Part model, mm, in its own coordinate system. Coordinates: 2 decimals unless noted, no trailing zeros. Loops run counter-clockwise (first coordinate to the right, second up) from the corner with the lowest first, then second, coordinate; pieces in that order, holes last. Notation, with made-up numbers: (-23, 21) -> (-1, 21) arc R32 cw to (-1, 55) -> close; hole circle Ø10 at (47.5, 43). An arc over 180 degrees is marked (long way). One line per question, with ' | ' between items. Start each with the question number.
1) Cut at B-B (z = 1.9). Count the separate pieces of the cut face and the enclosed holes in it, plus the area to 3 significant figures.
2) Cut at A-A (x = 20). List the corners of the cut face in (y, z), plus the area to 3 significant figures.
3) Drop flat-ended pins along their axis: pin 1 (1.3 mm diameter, centred on x = 147.5, z = 2.5, fed in from +Y); pin 2 (2 mm diameter, centred on y = 13, z = 3, fed in from +X); pin 3 (3 mm diameter, centred on x = -25.4, y = 7.62, fed in from +Z). Give the stop position or say it passes through.
4) Probe L1, parallel to X at y = 7.62, z = 2.35; L2, parallel to X at y = 83.5, z = 0.9; L3, parallel to X at y = 81, z = 1.6. List the from-to ranges inside material, lowest first. Write a range as from..to.
5) Cut at C-C (y = 34.5). List the corners of the cut face in (x, z), plus the area to 3 significant figures.
Autodesk Inventor part; units mm, degrees
ref_plane "YZ Plane" through (0, 0, 0) normal (1, 0, 0) x (0, 1, 0)
ref_plane "XZ Plane" through (0, 0, 0) normal (0, 1, 0) x (-1, 0, 0)
ref_plane "XY Plane" through (0, 0, 0) normal (0, 0, 1) x (1, 0, 0)
sketch "Sketch1" plane through (0, 0, 0) normal (0, 0, 1) x (1, 0, 0)
  line L0 (0, 105.156) -> (0, -17.526)
  line L1 (-209.804, 0) -> (209.804, 0)
  line L2 (101.6, 25.4) -> (-101.6, 25.4)
  line L3 (-101.6, 25.4) -> (-101.6, 0)
  line L4 (-101.6, 0) -> (101.6, 0)
  line L5 (101.6, 0) -> (101.6, 25.4)
  line L6 (101.6, 25.4) -> (-101.6, 0) construction
  line L7 (-101.6, 25.4) -> (101.6, 0) construction
  line L8 (149.86, 87.63) -> (-149.86, 87.63)
  line L9 (-149.86, 87.63) -> (-149.86, 25.4)
  line L10 (-149.86, 25.4) -> (149.86, 25.4)
  line L11 (149.86, 25.4) -> (149.86, 87.63)
  line L12 (149.86, 87.63) -> (-149.86, 25.4) construction
  line L13 (-149.86, 87.63) -> (149.86, 25.4) construction
  point P0 (0, 0)
  point P1 (0, 12.7)
  point P2 (0, 56.515)
  point P3 (-76.2, 7.62)
  point P4 (-25.4, 7.62)
  point P5 (25.4, 7.62)
  point P6 (76.2, 7.62)
  point P7 (-132.08, 79.8322)
  point P8 (132.08, 79.8322)
  point P9 (0, 79.8322)
  point P10 (-38.1, 79.8322)
  point P11 (38.1, 79.8322)
  dimension "d0" = 203.2
  dimension "d1" = 25.4
  dimension "d2" = 0
  dimension "d5" = 25.4
  dimension "d6" = 50.8
  dimension "d7" = 7.62
  dimension "d8" = 25.4
  dimension "d9" = 50.8
  dimension "d30" = 132.08
  dimension "d31" = 132.08
  dimension "d32" = 79.8322
  dimension "d33" = 87.63
  dimension "d34" = 299.72
  dimension "d62" = 38.1
  dimension "d63" = 38.1
extrude "Extrusion1" add sketch "Sketch1" along normal blind 4.4958
hole "Hole1" at (-76.2, 7.62, 0) at (-25.4, 7.62, 0) at (25.4, 7.62, 0) at (76.2, 7.62, 0) direction (0, 0, 1) diameter 3.1242 end through all
hole "Hole2" at (-132.08, 79.8322, 0) at (132.08, 79.8322, 0) at (0, 79.8322, 0) at (-38.1, 79.8322, 0) at (38.1, 79.8322, 0) direction (0, 0, 1) diameter 3.81 end through all
sketch "Sketch2" plane through (0, 0, 0) normal (0, 0, 1) x (1, 0, 0)
  circle A0 centre (132.08, 79.8322) radius 1.905
  circle A1 centre (-132.08, 79.8322) radius 1.905
  circle A2 centre (0, 79.8322) radius 1.905
  circle A3 centre (25.4, 7.62) radius 1.5621
  circle A4 centre (-76.2, 7.62) radius 1.5621
  circle A5 centre (-25.4, 7.62) radius 1.5621
  circle A6 centre (76.2, 7.62) radius 1.5621
  line L0 (-101.6, 25.4) -> (-101.6, 0)
  line L1 (-101.6, 0) -> (101.6, 0)
  line L2 (101.6, 0) -> (101.6, 25.4)
  line L3 (101.6, 25.4) -> (149.86, 25.4)
  line L4 (149.86, 25.4) -> (149.86, 87.63)
  line L5 (149.86, 87.63) -> (-149.86, 87.63)
  line L6 (-149.86, 87.63) -> (-149.86, 25.4)
  line L7 (-149.86, 25.4) -> (-101.6, 25.4)
  line L8 (-149.86, 87.63) -> (-137.16, 87.63)
  line L9 (-137.16, 87.63) -> (-137.16, 76.2)
  line L10 (-137.16, 76.2) -> (-149.86, 76.2)
  line L11 (-149.86, 76.2) -> (-149.86, 87.63)
  line L12 (149.86, 87.63) -> (137.16, 87.63)
  line L13 (137.16, 87.63) -> (137.16, 76.2)
  line L14 (137.16, 76.2) -> (149.86, 76.2)
  line L15 (149.86, 76.2) -> (149.86, 87.63)
  line L16 (-149.86, 87.63) -> (-149.2523, 87.63)
  line L17 (-149.2523, 87.63) -> (-151.5626, 87.63)
  line L18 (-151.5626, 87.63) -> (-149.86, 87.63)
  point P0 (0, 0)
  point P1 (-144.78, 67.945)
  point P2 (144.78, 67.945)
  point P3 (-138.43, 67.945)
  point P4 (138.43, 67.945)
  dimension "d35" = 11.43
  dimension "d36" = 12.7
  dimension "d39" = 8.255
  dimension "d40" = 5.08
  dimension "d41" = 5.08
  dimension "d64" = 6.35
  dimension "d65" = 6.35
extrude "Extrusion2" cut sketch "Sketch2" along normal up to next contours L6 L5 L9 L10 | L14 L13 L5 L4
hole "Hole3" at (-144.78, 67.945, 0) at (144.78, 67.945, 0) at (-138.43, 67.945, 0) at (138.43, 67.945, 0) direction (0, 0, 1) diameter 3.81 end through all
sketch "Sketch3" plane through (0, 0, 0) normal (0, 0, 1) x (1, 0, 0)
  line L0 (0, 105.156) -> (0, -17.526)
  line L1 (-209.804, 0) -> (209.804, 0)
  line L2 (137.16, 87.63) -> (-137.16, 87.63)
  line L3 (63.5, 83.058) -> (-63.5, 83.058)
  line L4 (-63.5, 83.058) -> (-63.5, 87.63)
  line L5 (-63.5, 87.63) -> (63.5, 87.63)
  line L6 (63.5, 87.63) -> (63.5, 83.058)
  line L7 (63.5, 83.058) -> (-63.5, 87.63) construction
  line L8 (-63.5, 83.058) -> (63.5, 87.63) construction
  point P0 (0, 0)
  point P1 (0, 85.344)
  dimension "d49" = 4.572
  dimension "d50" = 127
extrude "Extrusion3" cut sketch "Sketch3" along normal up to next
fillet "Fillet1" radius 6.35 2 edges at (-137.16, 76.2, 2.2479) (137.16, 76.2, 2.2479)
chamfer "Chamfer1" distance 38.1 angle 30 1 edges at (149.86, 25.4, 2.2479) measured on face at (117.6867, 25.4, 1.4986)
chamfer "Chamfer2" distance 38.1 angle 30 1 edges at (-149.86, 25.4, 2.2479) measured on face at (-133.7733, 25.4, 1.4986)
fillet "Fillet2" radius 12.7 4 edges at (-149.86, 47.397, 2.2479) (-111.76, 25.4, 2.2479) (111.76, 25.4, 2.2479) (149.86, 47.397, 2.2479)
fillet "Fillet3" radius 6.35 2 edges at (-101.6, 25.4, 2.2479) (101.6, 25.4, 2.2479)
properties material "DELRIN 100, BLACK (EXTRUDED)"
Reported:
1) separate pieces: 1 | enclosed holes: 13 | area: 22,000 mm²
2) outline: (0, 0) -> (83.06, 0) -> (83.06, 4.5) -> (0, 4.5) -> close | area: 373 mm²
3) pin 1: stops at y = 76.2 | pin 2: stops at x = 101.6 | pin 3: passes through
4) L1: x = -101.6..-77.76, -74.64..-26.96, -23.84..23.84, 26.96..74.64, 77.76..101.6 | L2: x = -137.16..-63.5, 63.5..137.16 | L3: x = -137.35..-133.59, -130.57..-39.61, -36.59..-1.51, 1.51..36.59, 39.61..130.57, 133.59..137.35
5) outline: (-127.52, 0) -> (127.52, 0) -> (127.52, 4.5) -> (-127.52, 4.5) -> close | area: 1,150 mm²
